Can you work these out from the drawing? Everything is in mm from the part's minimum corner. Coordinates: 2 decimals unless noted, no trailing zeros. Order: outer loops, then holes, each group sorted by start corner. A loop starts at its lowest first (then second) coordinate and runs counter-clockwise, first axis right, second up. Notation, with made-up numbers: (61.5, -38) -> (81.5, -38) arc R13 ccw to (81.5, -13) -> close; hole circle Ø9 at (6, 19). An arc over 180 degrees is marked (long way). Return JSON: item names as keys, results as strings. Group by question number.
1) If I drill on probe 1 along Y at (x, z) = (36.83, 7.5); probe 2 along Z at (x, y) = (59.5, 22); probe 3 along Y at (x, z) = (45.5, 17.5), over which ranges is the centre line in solid material (lowest first)? Write a range as from..to.
2) Thinking about a two-plate mould opening in X: for the marked faces 1, 2, 3 and 4, which applies, +X half, -X half, draft (parallel to the pull), parting line (faces both ways), or undercut?
3) If we section it at C-C, the plane z = 7.75: Please give me the cut outline in (x, y).
4) If we section it at A-A, the plane x = 36.83: Please give me the cut outline in (y, z).
5) For pin 1 (8 mm diameter, centred on x = 28.5, z = 4, fed in from +Y); pin 2 (5 mm diameter, centred on y = 40, z = 7, fed in from +X); pin 3 (8 mm diameter, centred on y = 55, z = 10.5, fed in from -X) (3 decimals), each with a flat end and sliding along its axis, tell me the tip position at first contact or that it passes through.
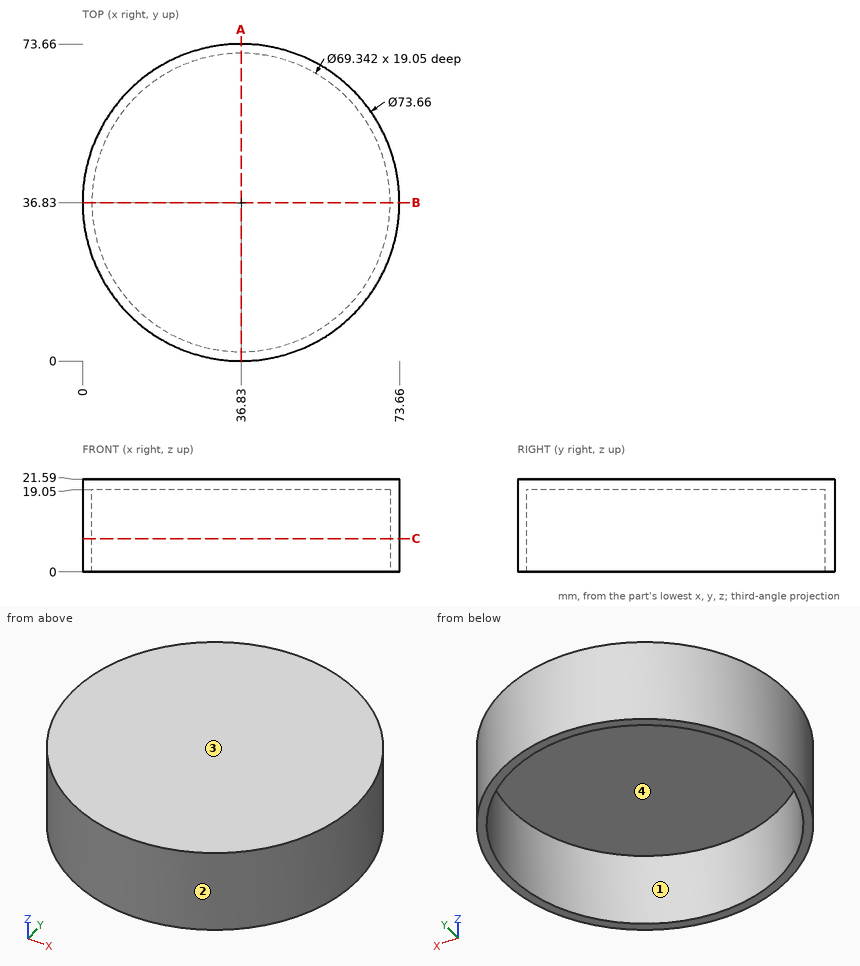
Result sheet:
{
 "1": {"probe 1": "y = 0..2.16, 71.5..73.66", "probe 2": "z = 19.05..21.59", "probe 3": "y = 1.04..3.26, 70.4..72.62"},
 "2": {"face 1": "undercut", "face 2": "parting line", "face 3": "draft", "face 4": "undercut"},
 "3": {"outline": "circle Ø73.66 at (36.83, 36.83); hole circle Ø69.34 at (36.83, 36.83)"},
 "4": {"outline": "(0, 0) -> (2.16, 0) -> (2.16, 19.05) -> (71.5, 19.05) -> (71.5, 0) -> (73.66, 0) -> (73.66, 21.59) -> (0, 21.59) -> close"},
 "5": {"pin 1": "stops at y = 73.4", "pin 2": "stops at x = 73.65", "pin 3": "stops at x = 2.835"}
}
